from build123d import *

# Parameters (mm, degrees)
F1_DEPTH  = 76.2
F2_W      = 12.7
F2_H      = 28.6385
F3_DEPTH  = 31.75
F5_DEPTH  = 50.8
F6_R      = 2.54
F7_R      = 2.54
F8_R      = 6.35
F9_R      = 2.38125
F10_DEPTH = 50.8
F12_DEPTH = 2.54
F14_DEPTH = 3.048


with BuildPart() as f1:
    # F0 (on Front) → F1 (new body)
    with BuildSketch(Plane.XZ):
        Polygon((22.2132794439, -11.7242682397), (22.2132794439, 16.9142317603), (-9.5367205561, 16.9142317603), (-9.5367205561, 10.5642317603), (9.5132794439, 10.5642317603), (9.5132794439, -5.3742682397), (-9.5367205561, -5.3742682397), (-9.5367205561, -11.7242682397), align=None)
    extrude(amount=F1_DEPTH)

    # F2 (on face) → F3 (join)
    with BuildSketch(Plane.YZ.offset(22.2132794439)):
        with Locations((-82.55, 2.5949817603)):
            Rectangle(F2_W, F2_H)
    extrude(amount=-F3_DEPTH)

    # F4 (on face) → F5 (join)
    with BuildSketch(Plane(origin=(-9.5367205561, 0, 0), x_dir=(0, -1, 0), z_dir=(-1, 0, 0))):
        Polygon((88.9, -11.7242682397), (88.9, 16.9142317603), (57.15, 16.9142317603), (57.15, 10.5642317603), (76.2, 10.5642317603), (76.2, -5.3742682397), (57.15, -5.3742682397), (57.15, -11.7242682397), align=None)
    extrude(amount=F5_DEPTH)

    # F6
    f6_edges = [f1.edges().sort_by_distance(p)[0] for p in [
        (-9.536721, -28.575, 16.914232),
    ]]
    fillet(f6_edges, radius=F6_R)

    # F7
    f7_edges = [f1.edges().sort_by_distance(p)[0] for p in [
        (-34.936721, -57.15, 16.914232),
    ]]
    fillet(f7_edges, radius=F7_R)

    # F8
    f8_edges = [f1.edges().sort_by_distance(p)[0] for p in [
        (22.213279, -88.9, 2.594982),
    ]]
    fillet(f8_edges, radius=F8_R)

    # F9 (on face) → F10 (cut)
    with BuildSketch(Plane.XY.offset(16.9142317603)):
        with Locations((1.2582794439, -67.945)):
            Circle(F9_R)
        with Locations((1.2582794439, -25.4)):
            Circle(F9_R)
        with Locations((-34.9367205561, -67.945)):
            Circle(F9_R)
    extrude(amount=-F10_DEPTH, mode=Mode.SUBTRACT)

    # F11 (on face) → F12 (join)
    with BuildSketch(Plane(origin=(-60.3367205561, 0, 0), x_dir=(0, -1, 0), z_dir=(-1, 0, 0))):
        Polygon((76.2, 13.7392317603), (76.2, 10.5642317603), (76.2, -5.3742682397), (76.2, -8.5492682397), (83.82, -8.5492682397), (83.82, 13.7392317603), align=None)
    extrude(amount=F12_DEPTH)

    # F13 (on face) → F14 (cut)
    with BuildSketch(Plane(origin=(0, 0, 0), x_dir=(-1, 0, 0), z_dir=(0, 1, 0))):
        Polygon((-8.7512794439, 14.5012317603), (-9.5132794439, 14.5012317603), (-17.8952794439, 14.5012317603), (-17.8952794439, -9.3112682397), (-9.5132794439, -9.3112682397), (-8.7512794439, -9.3112682397), (-8.7512794439, -5.3742682397), (-9.5132794439, -5.3742682397), (-9.5132794439, 10.5642317603), (-8.7512794439, 10.5642317603), align=None)
    extrude(amount=-F14_DEPTH, mode=Mode.SUBTRACT)


solid = f1.part
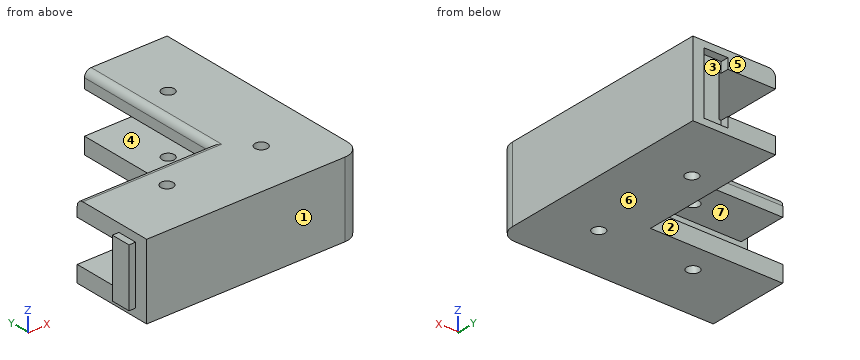
The listing builds one solid part. Answer for the finished solid, in the listing's coordinates (mm). Face numbers are marked on the shaded views. A direction names the side the tool comes from. Round coordinates to 2 decimals unless told otherwise and drop trailing zeros. Order: outer loops, then holes, each group sorted by start corner. A loop starts at its lowest first (then second) coordinate and runs counter-clockwise, first axis right, second up. Notation, with made-up numbers: (-8.75, 57.5) - (31.25, 57.5) arc R10 cw to (31.25, 72.5) - close; hole circle Ø5 at (89, -35.5). An arc over 180 degrees is marked (long way). Write item = value, one per line. Start each with the question number.
1) For a pull along Z with two mould halves and no side action, classify the marked faces 4, 5, 6 and 7 as released by +Z, released by -Z, zero draft, split by the parting line, or undercut.
2) Section C-C, the plane x = -47 is taken. Write down the section's boundary in (y, z), plus the area to 3 significant figures.
3) For the marked faces 1, 2 and 3, determine the directions among +Z, -Z, +X, -X, +Y, -Y from which every point of the face is accessible in a straight line to the end or side of a thin tool.
4) Section A-A, the plane y = -25.4 is taken. Write down the section's boundary in (x, z), plus the area to 3 significant figures.
5) Given pin 1 (4.5 mm diameter, centred on x = 1.26, y = -67.94, fed in from +Z); pin 2 (3 mm diameter, centred on y = -11, z = -7, fed in from -X); pin 3 (2 mm diameter, centred on x = -62, z = -2.5, fed in from -Y); pin 4 (12 mm diameter, centred on x = -5, z = 5, fed in from +Y), each flat-ended and moving along its own axis, determine where each tip first touches the part or whether it passes through.
6) Section B-B, the plane z = 2.25 is taken. Write down the section's boundary in (x, y), plus the area to 3 significant figures.
7) Straight lines are drawn through the part: L1, parallel to Z at x = 1, y = -52; L2, parallel to Y at x = -6.5, z = 0; L3, parallel to X at y = -46.5, z = -7.5. For each, find the intervals that lie inside material, in ascending order.
8) Section D-D, the plane y = -41 is taken. Write down the section's boundary in (x, z).
Results list:
q1.face_4 = undercut
q1.face_5 = zero draft
q1.face_6 = released by -Z
q1.face_7 = undercut
q2.outline = (-88.9, -11.72) - (-57.15, -11.72) - (-57.15, -5.37) - (-76.2, -5.37) - (-76.2, 10.56) - (-57.15, 10.56) - (-57.15, 14.37) arc R2.54 ccw to (-59.69, 16.91) - (-88.9, 16.91) - close
q2.area = 604 mm^2
q3.face_1 = +Z, -Z, +X, -X, -Y
q3.face_2 = +Z, -Z, -X, +Y
q3.face_3 = +Y
q4.outline = (-9.54, -11.72) - (-1.12, -11.72) - (-1.12, -5.37) - (-9.54, -5.37) - close; (-9.54, 10.56) - (-1.12, 10.56) - (-1.12, 16.91) - (-7, 16.91) arc R2.54 ccw to (-9.54, 14.37) - close; (3.64, -11.72) - (22.21, -11.72) - (22.21, 16.91) - (3.64, 16.91) - (3.64, 10.56) - (9.51, 10.56) - (9.51, -5.37) - (3.64, -5.37) - close
q4.area = 544 mm^2
q5.pin_1 = through
q5.pin_2 = -9.54
q5.pin_3 = -83.82
q5.pin_4 = 0
q6.outline = (-62.88, -83.82) - (-60.34, -83.82) - (-60.34, -88.9) - (15.86, -88.9) arc R6.35 ccw to (22.21, -82.55) - (22.21, 0) - (17.9, 0) - (17.9, -3.05) - (9.51, -3.05) - (9.51, -76.2) - (-62.88, -76.2) - close
q6.area = 2,000 mm^2
q7.L1 = -11.72 to -5.37, 10.56 to 16.91
q7.L2 = -88.9 to -76.2
q7.L3 = -9.54 to 22.21
q8.outline = (-9.54, -11.72) - (22.21, -11.72) - (22.21, 16.91) - (-7, 16.91) arc R2.54 ccw to (-9.54, 14.37) - (-9.54, 10.56) - (9.51, 10.56) - (9.51, -5.37) - (-9.54, -5.37) - close
